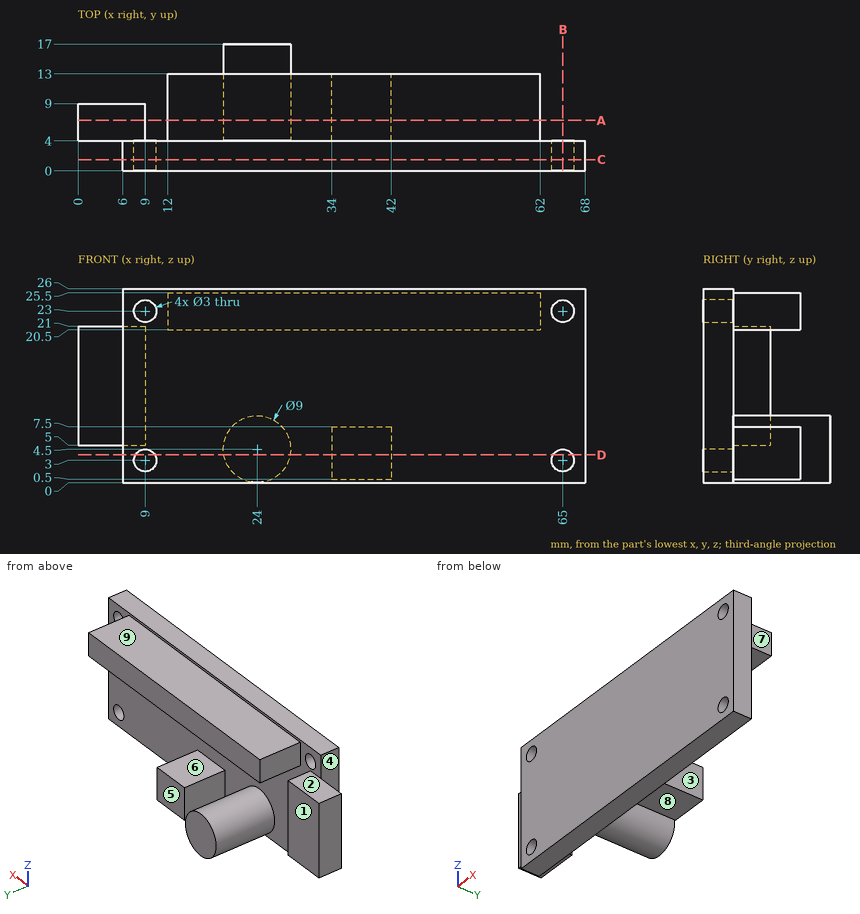
Geometry check sheet. Reference: drawing and pictorial views, mm from the part's lowest x, y, z. A direction names the side the tool comes from. Coordinates: 2 decimals unless noted, no trailing zeros. Loops run counter-clockwise (first coordinate to the right, second up) from the corner with the lowest first, then second, coordinate; pieces in that order, holes last. Notation, with made-up numbers: (19, 24.25) -> (66, 24.25) arc R25 ccw to (66, 39.25) -> close; hole circle Ø10 at (60.25, 13). An arc over 180 degrees is marked (long way). Put each result on its own line as item: value.
1) Tool access check on the marked faces 1, 2, 3, 4 and 5. Record the directions out of +Z, -Z, +X, -X, +Y, -Y that give a thin tool (end or side, any length) a straight path to the whole face; none if there is none.
Result set:
face 1: +Z, -Z, -X, +Y
face 2: +Z, -X, +Y
face 3: -Z, +X, +Y
face 4: +Z, -Z, -X, -Y
face 5: +Z, -Z, +X, +Y
2) Release check for a two-part mould opening along Z. For the marked faces 6, 7, 8 and 9 record: released by +Z, released by -Z, zero draft, split by the parting line, or undercut.
Result set:
face 6: undercut
face 7: zero draft
face 8: released by -Z
face 9: released by +Z
3) Cross-section at B-B on x = 65. Record the boundary of the cut face in (y, z).
Result set:
outline: (0, 0) -> (4, 0) -> (4, 1.5) -> (0, 1.5) -> close; (0, 4.5) -> (4, 4.5) -> (4, 21.5) -> (0, 21.5) -> close; (0, 24.5) -> (4, 24.5) -> (4, 26) -> (0, 26) -> close
4) Cross-section at C-C on y = 1.5. Record the boundary of the cut face in (x, z).
Result set:
outline: (6, 0) -> (68, 0) -> (68, 26) -> (6, 26) -> close; hole circle Ø3 at (9, 3); hole circle Ø3 at (9, 23); hole circle Ø3 at (65, 3); hole circle Ø3 at (65, 23)
5) Gauge pin test, flat ends, axial feed: pin 1 Ø8 at (x, y) = (43.5, 10.5) entering from -Z; pin 2 Ø2.5 at (x, y) = (6, 5.5) entering from -Z; pin 3 Ø4 at (x, z) = (12.5, 11) entering from +Y. Record the tip position at first contact, or that the pin passes through.
Result set:
pin 1: stops at z = 0.5
pin 2: stops at z = 5
pin 3: stops at y = 4
6) Cross-section at D-D on z = 3.75. Record the boundary of the cut face in (x, y), plus the area to 3 significant figures.
Result set:
outline: (6, 0) -> (7.7, 0) -> (7.7, 4) -> (6, 4) -> close; (10.3, 0) -> (63.7, 0) -> (63.7, 4) -> (42, 4) -> (42, 13) -> (34, 13) -> (34, 4) -> (28.44, 4) -> (28.44, 17) -> (19.56, 17) -> (19.56, 4) -> (10.3, 4) -> close; (66.3, 0) -> (68, 0) -> (68, 4) -> (66.3, 4) -> close
area: 415 mm^2
7) Thickness scan on line 1 (X direction, y = 1.3, z = 3); line 2 (Z direction, x = 65, y = 2.35); line 3 (X direction, y = 1, z = 2.5). Record the ranges inside material, lowest first.
Result set:
line 1: x = 6 to 7.5, 10.5 to 63.5, 66.5 to 68
line 2: z = 0 to 1.5, 4.5 to 21.5, 24.5 to 26
line 3: x = 6 to 7.59, 10.41 to 63.59, 66.41 to 68
8) Cross-section at A-A on y = 6.75. Record the boundary of the cut face in (x, z), plus the area to 3 significant figures.
Result set:
outline: (0, 5) -> (9, 5) -> (9, 21) -> (0, 21) -> close; (12, 20.5) -> (62, 20.5) -> (62, 25.5) -> (12, 25.5) -> close; circle Ø9 at (24, 4.5); (34, 0.5) -> (42, 0.5) -> (42, 7.5) -> (34, 7.5) -> close
area: 514 mm^2
